```python
from build123d import *

# Parameters (mm, degrees)
SALIENTE_EXTRUIR1_DEPTH = 4


with BuildPart() as part:
    # Croquis1 → Saliente-Extruir1 (new body)
    with BuildSketch(Plane(origin=(0, 0, 0), x_dir=(0, 0, -1), z_dir=(1, 0, 0))):
        Polygon((-81, -25), (-81, -29), (-51, -29), (-51, -25), (51, -25), (51, -29), (81, -29), (81, -25), (90.8, -25), (90.8, 25), (20, 25), (20, 35), (-20, 35), (-20, 25), (-90.8, 25), (-90.8, -25), align=None)
        with BuildLine():
            Line((-50, 16.519823789), (50, 16.519823789))
            ThreePointArc((50, 16.519823789), (57.071067812, 13.5908916), (60, 6.519823789))
            Line((60, 6.519823789), (60, -6.519823789))
            ThreePointArc((60, -6.519823789), (57.071067812, -13.5908916), (50, -16.519823789))
            Line((50, -16.519823789), (-50, -16.519823789))
            ThreePointArc((-50, -16.519823789), (-57.071067812, -13.5908916), (-60, -6.519823789))
            Line((-60, -6.519823789), (-60, 6.519823789))
            ThreePointArc((-60, 6.519823789), (-57.071067812, 13.5908916), (-50, 16.519823789))
        make_face(mode=Mode.SUBTRACT)
    extrude(amount=SALIENTE_EXTRUIR1_DEPTH)


solid = part.part
```
Input: part model. Units: mm. Frame: model coordinates. A direction names the side the tool comes from. Give positions to 0.01 mm unless a question says otherwise; leave off trailing zeros. Order: outer loops, then holes, each group sorted by start corner. A loop starts at its lowest first (then second) coordinate and runs counter-clockwise, first axis right, second up. Notation, with made-up numbers: M 73.25,-4 L 113.25,-4 A18 ccw 113.25,16 Z; hole C -39,47 d1. An arc over 180 degrees is marked long. One line per question, with ' | ' between items.
1) Draft query along Z for faces 4 (the face through (2, 25, 55)), 5 (the face through (2, -27, -81)), 6 (the face through (2, 0, -60)), 7 (the face through (1.97, -13.51, -57.15)). Return one class per face: pulls with the +Z half, pulls with the -Z half, needs draft (parallel to the pull), parting line crosses it, or undercut.
Filled in:
face 4: needs draft | face 5: pulls with the -Z half | face 6: undercut | face 7: undercut
2) Section A-A on z = 25.5. Output: boundary loops of the cut face in (x, y).
Filled in:
outline: M 0,-25 L 4,-25 L 4,-16.52 L 0,-16.52 Z; M 0,16.52 L 4,16.52 L 4,25 L 0,25 Z
3) Ray query, L1, parallel to Y at x = 3.7, z = -33.5; L2, parallel to Z at x = 1.15, y = -6; L3, parallel to Y at x = 0.8, z = -18. Return the intervals inside material, ascending.
Filled in:
L1: y = -25 to -16.52, 16.52 to 25 | L2: z = -90.8 to -60, 60 to 90.8 | L3: y = -25 to -16.52, 16.52 to 35
4) Access query for faces 1 (the face through (2, 25, -56)), 2 (the face through (2, -27, -51)), 3 (the face through (1.97, 13.67, -56.99)). Directions: +Z, -Z, +X, -X, +Y, -Y. A direction counts if a zero-diameter tool reaches every point of the face in a straight line with its end or side. Return the directions, or none.
Filled in:
face 1: -Z, +X, -X, +Y | face 2: +X, -X, -Y | face 3: +X, -X
5) Section C-C on x = 2.3. Output: boundary loops of the cut face in (y, z), and give its area (3 significant figures).
Filled in:
outline: M -29,-81 L -25,-81 L -25,-90.8 L 25,-90.8 L 25,-20 L 35,-20 L 35,20 L 25,20 L 25,90.8 L -25,90.8 L -25,81 L -29,81 L -29,51 L -25,51 L -25,-51 L -29,-51 Z; hole M -16.52,-50 A10 ccw -6.52,-60 L 6.52,-60 A10 ccw 16.52,-50 L 16.52,50 A10 ccw 6.52,60 L -6.52,60 A10 ccw -16.52,50 Z | area: 5,840 mm2
6) Section D-D on y = 29.5. Output: boundary loops of the cut face in (x, z).
Filled in:
outline: M 0,-20 L 4,-20 L 4,20 L 0,20 Z
7) Contact query for flat-ended pins moving along their axis: P1, Ø1.2, axis at x = 1, y = 29.5, coming from the +Z side; P2, Ø1.2, axis at x = 2.5, z = -84.5, coming from the -Y side; P3, Ø2, axis at x = 1.5, y = -27.5, coming from the -Z side. Output: stop coordinate, or through.
Filled in:
P1: stops at z = 20 | P2: stops at y = -25 | P3: stops at z = -81
8) Section B-B on y = 4.5. Output: boundary loops of the cut face in (x, z), and give its area (3 significant figures).
Filled in:
outline: M 0,-90.8 L 4,-90.8 L 4,-60 L 0,-60 Z; M 0,60 L 4,60 L 4,90.8 L 0,90.8 Z | area: 246 mm2
